Can you work these out from the model? Positions are in its coordinate system, mm. A direction names the side the tool comes from. Give positions to 0.01 mm unless a question says otherwise; leave off trailing zeros. Loops run counter-clockwise (first coordinate to the right, second up) from the corner with the lowest first, then second, coordinate; pieces in that order, holes last. Notation, with made-up numbers: (12.5, 71.5) - (69.5, 71.5) arc R22 ccw to (69.5, 101.5) - close; hole circle Ø5 at (27, 63.25). An arc over 180 degrees is marked (long way). Answer as a JSON object with one key per item and string values.
```python
from build123d import *

# Parameters (mm, degrees)
SKETCH1_W          = 38.1
SKETCH1_H          = 76.2
SKETCH1_R          = 4.1656
SKETCH1_R_2        = 4.7625
EXTRUDE1_DEPTH     = 19.05
SKETCH2_R          = 6.5405
CUT_EXTRUDE1_DEPTH = 8.128
CHAMFER1_SIZE      = 0.254


with BuildPart() as part:
    # Sketch1 → Extrude1 (new body)
    with BuildSketch(Plane(origin=(0, 0, 0), x_dir=(1, 0, 0), z_dir=(0, 1, 0))):
        with Locations((-6.35, 38.1)):
            Rectangle(SKETCH1_W, SKETCH1_H)
        with Locations(Location((-6.35, 57.15, 0), (0, 0, 90))):
            Circle(SKETCH1_R, mode=Mode.SUBTRACT)
        with Locations(Location((-6.35, 19.05, 0), (0, 0, 90))):
            Circle(SKETCH1_R, mode=Mode.SUBTRACT)
        with Locations(Location((-6.35, 38.1, 0), (0, 0, 90))):
            Circle(SKETCH1_R_2, mode=Mode.SUBTRACT)
    extrude(amount=EXTRUDE1_DEPTH)

    # Sketch2 → Cut-Extrude1 (cut)
    with BuildSketch(Plane(origin=(0, 19.05, 0), x_dir=(1, 0, 0), z_dir=(0, 1, 0))):
        with Locations(Location((-6.35, 57.15, 0), (0, 0, 270))):
            Circle(SKETCH2_R)
        with Locations(Location((-6.35, 19.05, 0), (0, 0, 270))):
            Circle(SKETCH2_R)
    extrude(amount=-CUT_EXTRUDE1_DEPTH, mode=Mode.SUBTRACT)

    # Chamfer1
    chamfer1_edges = [part.edges().sort_by_distance(p)[0] for p in [
        (12.7, 19.05, -38.1),
        (-6.35, 19.05, -76.2),
        (-25.4, 19.05, -38.1),
        (-6.35, 0, -76.2),
        (12.7, 0, -38.1),
        (-6.35, 0, 0),
        (-25.4, 0, -38.1),
        (-6.35, 19.05, 0),
        (-25.4, 9.525, -76.2),
        (12.7, 9.525, -76.2),
        (12.7, 9.525, 0),
        (-25.4, 9.525, 0),
    ]]
    chamfer(chamfer1_edges, length=CHAMFER1_SIZE)


solid = part.part
```
1) Imagine slicing it at D-D on z = -19.05. Write out the boundary of the cut face in (x, y), and give its area (3 significant figures).
Check sheet entries:
{"outline": "(-25.4, 0.25) - (-25.15, 0) - (-10.52, 0) - (-10.52, 10.92) - (-12.89, 10.92) - (-12.89, 19.05) - (-25.15, 19.05) - (-25.4, 18.8) - close; (-2.18, 0) - (12.45, 0) - (12.7, 0.25) - (12.7, 18.8) - (12.45, 19.05) - (0.19, 19.05) - (0.19, 10.92) - (-2.18, 10.92) - close", "area": "528 mm2"}
2) I'm going to push flat-ended pins straight in: P1, Ø11, axis at x = -6.35, z = -38.1, coming from the +Y side; P2, Ø11, axis at x = -6.35, z = -57.15, coming from the +Y side. Where does each tip first touch, or does it pass through?
Check sheet entries:
{"P1": "y = 19.05", "P2": "y = 10.92"}
3) I need wall thicknesses on L1, parallel to X at y = 8.75, z = -19.05; L2, parallel to Z at x = -5, y = 14; L3, parallel to Z at x = -4, y = 12.5. Which ranges of each line are inside material? Lowest first, please.
Check sheet entries:
{"L1": "-25.4 to -10.52, -2.18 to 12.7", "L2": "-76.2 to -63.55, -50.75 to -42.67, -33.53 to -25.45, -12.65 to 0", "L3": "-76.2 to -63.25, -51.05 to -42.24, -33.96 to -25.15, -12.95 to 0"}
4) Imagine slicing it at C-C on y = 12. Give the number of separate pieces and of enclosed holes in the cut face, and give its area (3 significant figures).
Check sheet entries:
{"separate pieces": "1", "enclosed holes": "3", "area": "2,560 mm2"}
5) If we mould it in two halves opening along X, with no side actions, what happens to faces 1 (the flat face through (-7, 19.05, -47)), 2 (the flat face through (-25.4, 9, -38)), 3 (the cylindrical face through (-3.82, 5.38, -15.74)), 4 (the cylindrical face through (-6.062, 15.043, -25.584))? For each: released by +X, released by -X, zero draft, split by the parting line, or undercut.
Check sheet entries:
{"face 1": "zero draft", "face 2": "released by -X", "face 3": "undercut", "face 4": "undercut"}
6) Imagine slicing it at A-A on z = -38.1. Write out the boundary of the cut face in (x, y), and give its area (3 significant figures).
Check sheet entries:
{"outline": "(-25.4, 0.25) - (-25.15, 0) - (-11.11, 0) - (-11.11, 19.05) - (-25.15, 19.05) - (-25.4, 18.8) - close; (-1.59, 0) - (12.45, 0) - (12.7, 0.25) - (12.7, 18.8) - (12.45, 19.05) - (-1.59, 19.05) - close", "area": "544 mm2"}
7) Which directions (+Z, -Z, +X, -X, +Y, -Y) give clear straight access to the entire face, cutting with the end or side of a thin tool? Please do faces 5 (the flat face through (12.7, 9, -38)), 6 (the flat face through (-11, 10.922, -57)).
Check sheet entries:
{"face 5": "+Z, -Z, +X, +Y, -Y", "face 6": "+Y"}
8) Imagine slicing it at B-B on x = -6.35. Write out the boundary of the cut face in (y, z).
Check sheet entries:
{"outline": "(0, -75.95) - (0.25, -76.2) - (18.8, -76.2) - (19.05, -75.95) - (19.05, -63.69) - (10.92, -63.69) - (10.92, -61.32) - (0, -61.32) - close; (0, -52.98) - (10.92, -52.98) - (10.92, -50.61) - (19.05, -50.61) - (19.05, -42.86) - (0, -42.86) - close; (0, -33.34) - (19.05, -33.34) - (19.05, -25.59) - (10.92, -25.59) - (10.92, -23.22) - (0, -23.22) - close; (0, -14.88) - (10.92, -14.88) - (10.92, -12.51) - (19.05, -12.51) - (19.05, -0.25) - (18.8, 0) - (0.25, 0) - (0, -0.25) - close"}
